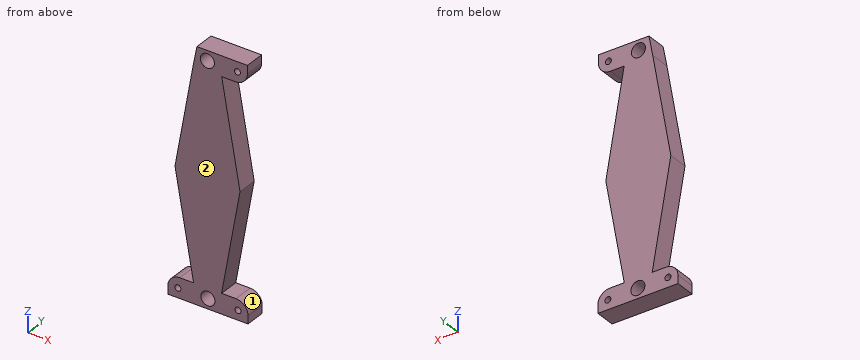
from build123d import *

# Parameters (mm, degrees)
SKETCH2_R           = 1.5
SKETCH2_R_2         = 3.5
SKETCH2_W           = 40
SKETCH2_H           = 10
BOSS_EXTRUDE1_DEPTH = 10
FILLET1_R           = 6
CUT_EXTRUDE2_DEPTH  = 11


with BuildPart() as part:
    # Sketch2 → Boss-Extrude1 (new body)
    with BuildSketch(Plane(origin=(0, 0, 0), x_dir=(1, 0, 0), z_dir=(0, 1, 0))):
        Polygon((27.08938228, 113.93955974), (13.128576505, 113.93955974), (3.831784068, 61.214829812), (12.862340376, 10), (27.137659624, 10), (36.277195325, 61.83288266), align=None)
        Polygon((0.266236129, 113.93955974), (13.128576505, 113.93955974), (27.08938228, 113.93955974), (40.266236129, 113.93955974), (40.266236129, 123.93955974), (0.266236129, 123.93955974), align=None)
        with Locations((5.266236129, 119.206649777)):
            Circle(SKETCH2_R, mode=Mode.SUBTRACT)
        with Locations((20.266236129, 118.93955974)):
            Circle(SKETCH2_R_2, mode=Mode.SUBTRACT)
        with Locations((35.266236129, 119.206649777)):
            Circle(SKETCH2_R, mode=Mode.SUBTRACT)
        with Locations((20, 5)):
            Rectangle(SKETCH2_W, SKETCH2_H)
        with Locations((35, 4.874301968)):
            Circle(SKETCH2_R, mode=Mode.SUBTRACT)
        with Locations((5, 4.874301968)):
            Circle(SKETCH2_R, mode=Mode.SUBTRACT)
        with Locations((20, 5)):
            Circle(SKETCH2_R_2, mode=Mode.SUBTRACT)
    extrude(amount=BOSS_EXTRUDE1_DEPTH)

    # Fillet1
    fillet1_edges = [part.edges().sort_by_distance(p)[0] for p in [
        (40, 5, -10),
        (0, 5, -10),
        (0.266236129, 5, -113.93955974),
        (40.266236129, 5, -113.93955974),
    ]]
    fillet(fillet1_edges, radius=FILLET1_R)

    # Sketch3 → Cut-Extrude2 (cut, through all)
    with BuildSketch(Plane(origin=(0, 10, 0), x_dir=(1, 0, 0), z_dir=(0, 1, 0))):
        Polygon((14.761999195, 0), (0, 0), (0, 10.134747314), (12.862340376, 10), align=None)
    extrude(amount=-CUT_EXTRUDE2_DEPTH, mode=Mode.SUBTRACT)


solid = part.part
Design review of the part built by this model. Coordinates are the model's own, in mm. Face numbers are marked on the shaded views. Round coordinates to 2 decimals unless told otherwise and drop trailing zeros. Loops run counter-clockwise (first coordinate to the right, second up) from the corner with the lowest first, then second, coordinate; pieces in that order, holes last. Notation, with made-up numbers: (33.5, 78) -> (65.5, 78) arc R29 cw to (65.5, 100) -> close; hole circle Ø7 at (65, 44.5). An arc over 180 degrees is marked (long way). Use one line per item in the form item = value. Start each with the question number.
Q1. Draft analysis for pull direction X (two halves, no side actions). For the marked faces 1 and 2, state which applies: +X half, -X half, draft (parallel to the pull), parting line (faces both ways), or undercut.
Q2. For pin 1 Ø6.5 at (x, z) = (20, -5) entering from +Y; pin 2 Ø6 at (y, z) = (8, -88.5) entering from -X; pin 3 Ø3 at (y, z) = (5, -2.5) entering from +X, all flat-tipped, find the tip position at first contact; note any pin that passes through.
Q3. We need section C-C on z = -50.5. Give the boundary of the cut face in (x, y).
Q4. Wall thickness on line 1 along Z through (x, y) = (20, 4.25); line 2 along Z through (x, y) = (18.5, 8); line 3 along Z through (x, y) = (37.5, 4): over which ranges is each line inside the solid? List them lowest first. Write a range as [from, to].
Q5. We need section D-D on z = -86.5. Give the boundary of the cut face in (x, y).
Q6. We need section A-A on x = 20. Give the boundary of the cut face in (y, z).
Q7. We need section B-B on y = 2.5. Give the boundary of the cut face in (x, z).
Calculated:
q1.face_1 = +X half
q1.face_2 = draft
q2.pin_1 = through
q2.pin_2 = 8.11
q2.pin_3 = 40
q3.outline = (5.72, 0) -> (34.28, 0) -> (34.28, 10) -> (5.72, 10) -> close
q4.line_1 = [-123.94, -122.43], [-115.45, -8.5], [-1.5, 0]
q4.line_2 = [-123.94, -121.96], [-115.92, -8.16], [-1.84, 0]
q4.line_3 = [-123.94, -114.89], [-8.87, 0]
q5.outline = (8.29, 0) -> (31.93, 0) -> (31.93, 10) -> (8.29, 10) -> close
q6.outline = (0, -123.94) -> (10, -123.94) -> (10, -122.43) -> (0, -122.43) -> close; (0, -115.45) -> (10, -115.45) -> (10, -8.5) -> (0, -8.5) -> close; (0, -1.5) -> (10, -1.5) -> (10, 0) -> (0, 0) -> close
q7.outline = (0.27, -123.94) -> (40.27, -123.94) -> (40.27, -119.94) arc R6 ccw to (34.27, -113.94) -> (27.09, -113.94) -> (36.28, -61.83) -> (27.14, -10) -> (34, -10) arc R6 ccw to (40, -4) -> (40, 0) -> (14.76, 0) -> (12.86, -10) -> (3.83, -61.21) -> (13.13, -113.94) -> (6.27, -113.94) arc R6 ccw to (0.27, -119.94) -> close; hole circle Ø3 at (5.27, -119.21); hole circle Ø7 at (20, -5); hole circle Ø7 at (20.27, -118.94); hole circle Ø3 at (35, -4.87); hole circle Ø3 at (35.27, -119.21)
